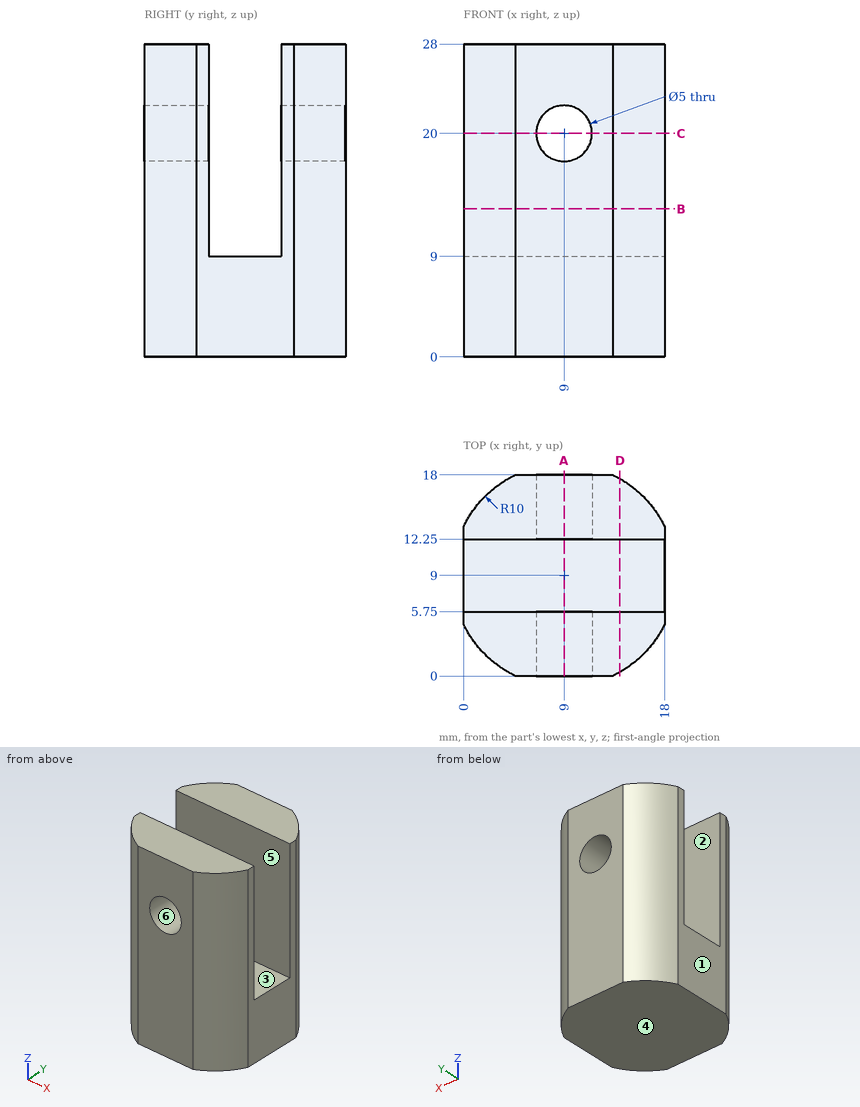
Part print with two shaded views. Sizes in mm from the minimum x, y, z corner. A direction names the side the tool comes from. Round coordinates to 2 decimals unless told otherwise and drop trailing zeros. Order: outer loops, then holes, each group sorted by start corner. A loop starts at its lowest first (then second) coordinate and runs counter-clockwise, first axis right, second up. Notation, with made-up numbers: M -33,6.5 L -27,6.5 A13 cw -27,19.5 Z; hole C 1,25.5 d10. An arc over 180 degrees is marked long. Use CSV: the item, a comma, the result in double quotes.
Item 1: Saw through at C-C (z = 20). List the corners of the cut face in (x, y).
Worked answers:
outline,"M 0,4.64 A10 ccw 4.64,0 L 6.5,0 L 6.5,5.75 L 0,5.75 Z; M 0,12.25 L 6.5,12.25 L 6.5,18 L 4.64,18 A10 ccw 0,13.36 Z; M 11.5,0 L 13.36,0 A10 ccw 18,4.64 L 18,5.75 L 11.5,5.75 Z; M 11.5,12.25 L 18,12.25 L 18,13.36 A10 ccw 13.36,18 L 11.5,18 Z"
Item 2: Which spindle directions (+Z, -Z, +X, -X, +Y, -Y) get a long thin tool onto all of the face, cutting with end or side? Do the marked faces 1 and 2. Say none if no direction does.
Worked answers:
face 1,"+Z, -Z, -X, +Y, -Y"
face 2,"+Z, +X, -X"
Item 3: Saw through at B-B (z = 13.25). List the corners of the cut face in (x, y).
Worked answers:
outline,"M 0,4.64 A10 ccw 4.64,0 L 13.36,0 A10 ccw 18,4.64 L 18,5.75 L 0,5.75 Z; M 0,12.25 L 18,12.25 L 18,13.36 A10 ccw 13.36,18 L 4.64,18 A10 ccw 0,13.36 Z"
Item 4: Pull direction Z, two halves, no side cores. Call the marked faces 3, 4, 5 and 6: released by +Z, released by -Z, zero draft, split by the parting line, or undercut.
Worked answers:
face 3,"released by +Z"
face 4,"released by -Z"
face 5,"zero draft"
face 6,"undercut"
Item 5: Pin check, flat tip, straight feed: pin 1 (5 mm diameter, centred on x = 8, y = 9, fed in from +Z). Stop position of the tip, or through.
Worked answers:
pin 1,"z = 9"
Item 6: Probe probe 1 along Z at (x, y) = (9, 14.8); probe 2 along Y at (x, z) = (9.75, 17.25); probe 3 along Z at (x, y) = (16.5, 11.5). List the from-to ranges inside material, lowest first.
Worked answers:
probe 1,"0 to 17.5, 22.5 to 28"
probe 2,"0 to 5.75, 12.25 to 18"
probe 3,"0 to 9"
Item 7: Saw through at A-A (x = 9). List the corners of the cut face in (y, z).
Worked answers:
outline,"M 0,0 L 18,0 L 18,17.5 L 12.25,17.5 L 12.25,9 L 5.75,9 L 5.75,17.5 L 0,17.5 Z; M 0,22.5 L 5.75,22.5 L 5.75,28 L 0,28 Z; M 12.25,22.5 L 18,22.5 L 18,28 L 12.25,28 Z"
Item 8: Saw through at D-D (x = 14). List the corners of the cut face in (y, z), plus the area to 3 significant figures.
Worked answers:
outline,"M 0.34,0 L 17.66,0 L 17.66,28 L 12.25,28 L 12.25,9 L 5.75,9 L 5.75,28 L 0.34,28 Z"
area,"361 mm²"
